Check sheet for the modelled part. Datum: model origin and axes. Units: mm. Give positions to 0.01 mm unless a question says otherwise; leave off trailing zeros. Write each loop counter-clockwise with the first axis right and the second up, starting at its lowest first coordinate (ties: lowest second). Pieces come first, ordered by that corner, then holes. Notation, with made-up numbers: (-6.75, 70.25) -> (-2.75, 70.25) arc R20 ccw to (-2.75, 97.25) -> close; hole circle Ø2 at (48, -19.5). An arc over 180 degrees is marked (long way). Use a Markdown table: item, result. Add a question column.
1. Cross-section at A-A (x = 25). Enter the section's corners in (y, z).
2. Cross-section at C-C (z = 2.05). Enter the section's corners in (x, y).
3. Gauge pin test, flat end, axial feed: P1, Ø1.5, axis at y = 20.5, z = 2.5, coming from the -X side. Record the tip position at first contact, or that the pin passes through.
4. Cross-section at D-D (y = 45). Enter the section's corners in (x, z), then the cut area to 4 significant figures.
5. Scan lines: probe 1 along Y at (x, z) = (25, 2); probe 2 along X at (y, z) = (8.5, 2.4); probe 3 along Y at (x, z) = (61, 2). Record each from-to range of solid material in increasing order. Write a range as [from, to].
6. Cross-section at B-B (y = 10). Enter the section's corners in (x, z), then the cut area to 4 significant figures.
from build123d import *

# Parameters (mm, degrees)
F0_R     = 2.5
F1_DEPTH = 3


with BuildPart() as f1:
    # F0 (on Top) → F1 (new body)
    with BuildSketch(Plane.XY):
        with BuildLine():
            Line((0, 18.81966), (0, 5))
            ThreePointArc((0, 5), (1.464466, 1.464466), (5, 0))
            Line((5, 0), (62.5, 0))
            ThreePointArc((62.5, 0), (66.035534, 1.464466), (67.5, 5))
            Line((67.5, 5), (67.5, 17.810844))
            ThreePointArc((67.5, 17.810844), (67.080229, 19.816211), (65.891401, 21.484861))
            Line((65.891401, 21.484861), (36.436481, 48.674017))
            ThreePointArc((36.436481, 48.674017), (34.865783, 49.65672), (33.045081, 50))
            Line((33.045081, 50), (18.09017, 50))
            ThreePointArc((18.09017, 50), (15.461514, 49.253254), (13.618034, 47.236068))
            Line((13.618034, 47.236068), (0.527864, 21.055728))
            ThreePointArc((0.527864, 21.055728), (0.133755, 19.968425), (0, 18.81966))
        make_face()
        with Locations((5, 10)):
            Circle(F0_R, mode=Mode.SUBTRACT)
        with Locations((25, 10)):
            Circle(F0_R, mode=Mode.SUBTRACT)
        with Locations((62.5, 10)):
            Circle(F0_R, mode=Mode.SUBTRACT)
        with Locations((25, 30)):
            Circle(F0_R, mode=Mode.SUBTRACT)
        with Locations((25, 45)):
            Circle(F0_R, mode=Mode.SUBTRACT)
    extrude(amount=F1_DEPTH)


solid = f1.part
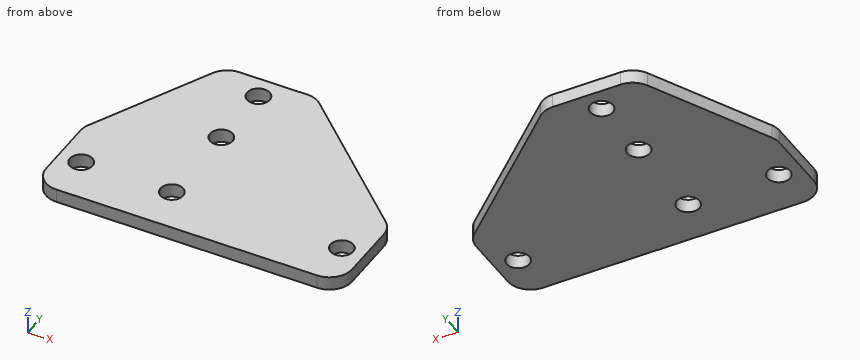
Worked answers:
| question | item | result |
|---|---|---|
| 1 | outline | (0, 0) -> (7.5, 0) -> (7.5, 3) -> (0, 3) -> close; (12.5, 0) -> (27.5, 0) -> (27.5, 3) -> (12.5, 3) -> close; (32.5, 0) -> (42.5, 0) -> (42.5, 3) -> (32.5, 3) -> close; (47.5, 0) -> (50, 0) -> (50, 3) -> (47.5, 3) -> close |
| 2 | outline | (0, 5) arc R5 ccw to (5, 0) -> (62.5, 0) arc R5 ccw to (67.5, 5) -> (67.5, 17.81) arc R5 ccw to (65.89, 21.48) -> (36.44, 48.67) arc R5 ccw to (33.05, 50) -> (18.09, 50) arc R5 ccw to (13.62, 47.24) -> (0.53, 21.06) arc R5 ccw to (0, 18.82) -> close; hole circle Ø5 at (5, 10); hole circle Ø5 at (25, 10); hole circle Ø5 at (25, 30); hole circle Ø5 at (25, 45); hole circle Ø5 at (62.5, 10) |
| 3 | P1 | stops at x = 0.09 |
| 4 | outline | (12.5, 0) -> (22.5, 0) -> (22.5, 3) -> (12.5, 3) -> close; (27.5, 0) -> (40.42, 0) -> (40.42, 3) -> (27.5, 3) -> close |
| 4 | area | 68.75 mm² |
| 5 | probe 1 | y = [0, 7.5], [12.5, 27.5], [32.5, 42.5], [47.5, 50] |
| 5 | probe 2 | x = [0, 3], [7, 23], [27, 60.5], [64.5, 67.5] |
| 5 | probe 3 | y = [0, 8], [12, 26] |
| 6 | outline | (0, 0) -> (2.5, 0) -> (2.5, 3) -> (0, 3) -> close; (7.5, 0) -> (22.5, 0) -> (22.5, 3) -> (7.5, 3) -> close; (27.5, 0) -> (60, 0) -> (60, 3) -> (27.5, 3) -> close; (65, 0) -> (67.5, 0) -> (67.5, 3) -> (65, 3) -> close |
| 6 | area | 157.5 mm² |
